Design review of the part built by this model. Coordinates are the model's own, in mm. Face numbers are marked on the shaded views. Coordinates: 2 decimals unless noted, no trailing zeros. Loops run counter-clockwise (first coordinate to the right, second up) from the corner with the lowest first, then second, coordinate; pieces in that order, holes last. Notation, with made-up numbers: M -32,-31 L -12,-31 A27 ccw -12,2 Z; hole C 39.5,84 d9. An arc over 180 degrees is marked long. Answer as a JSON object with one key per item and string values. Group by question number.
1. Consider section A-A (y = 0). State the section outline as (x, z) points, then the cut area to 3 significant figures.
2. To check wall thickness, follow probe 1 along Z at (x, y) = (-6, 2); probe 2 along Y at (x, z) = (-3.5, 5.75); probe 3 along Y at (x, z) = (14, 7). State the ranges of each line that lie inside material, in increasing order.
3. Insertion check: pin 1 (1.5 mm diameter, centred on x = -5, z = 3.5, fed in from +Y); pin 2 (1.5 mm diameter, centred on y = 13, z = 6.5, fed in from +X); pin 3 (2 mm diameter, centred on y = -12, z = 3, fed in from +X). Each pin has a flat end and moves straight along its axis. Give the tip position at first contact, or say it passes through.
4. Consider section C-C (z = 3.5). State the section outline as (x, y) points.
5. Draft analysis for pull direction Y (two halves, no side actions). For the marked faces 1, 2, 3 and 4, state which applies: +Y half, -Y half, draft (parallel to the pull), parting line (faces both ways), or undercut.
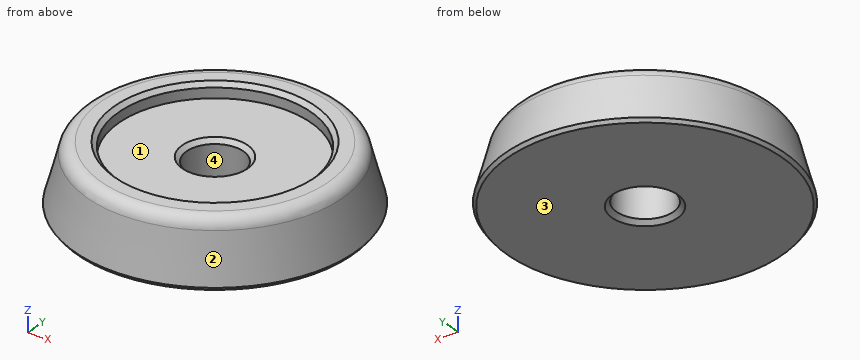
from build123d import *

# Parameters (mm, degrees)
F2_SIZE = 0.6
F3_R    = 2
F4_SIZE = 0.5


with BuildPart() as f1:
    # F0 (on Front) → F1 (revolve)
    with BuildSketch(Plane.XZ):
        Polygon((4, 6.5), (4, 0), (19.777568, 0), (17.5, 8.5), (13.5, 8.5), (13.5, 6.5), align=None)
    revolve(axis=Axis((0, 0, 2.242119), (0, 0, 1)))

    # F2
    f2_edges = [f1.edges().sort_by_distance(p)[0] for p in [
        (-13.5, 0, 8.5),
        (-4, 0, 6.5),
        (-4, 0, 0),
    ]]
    chamfer(f2_edges, length=F2_SIZE)

    # F3
    f3_edges = [f1.edges().sort_by_distance(p)[0] for p in [
        (-17.5, 0, 8.5),
    ]]
    fillet(f3_edges, radius=F3_R)

    # F4
    f4_edges = [f1.edges().sort_by_distance(p)[0] for p in [
        (-19.777568, 0, 0),
    ]]
    chamfer(f4_edges, length=F4_SIZE)


solid = f1.part
Findings below:
{
 "1": {"outline": "M -19.65,0.48 L -19.28,0 L -4.6,0 L -4,0.6 L -4,5.9 L -4.6,6.5 L -13.5,6.5 L -13.5,7.9 L -14.1,8.5 L -15.97,8.5 A2 ccw -17.9,7.02 Z; M 4,0.6 L 4.6,0 L 19.28,0 L 19.65,0.48 L 17.9,7.02 A2 ccw 15.97,8.5 L 14.1,8.5 L 13.5,7.9 L 13.5,6.5 L 4.6,6.5 L 4,5.9 Z", "area": "209 mm^2"},
 "2": {"probe 1": "z = 0 to 6.5", "probe 2": "y = -17.9 to -1.94, 1.94 to 17.9", "probe 3": "y = -11.16 to 11.16"},
 "3": {"pin 1": "stops at y = 18.45", "pin 2": "stops at x = 13.29", "pin 3": "stops at x = 15.53"},
 "4": {"outline": "C 0,0 d37.68; hole C 0,0 d8"},
 "5": {"face 1": "undercut", "face 2": "parting line", "face 3": "draft", "face 4": "undercut"}
}
